```python
from build123d import *

# Parameters (mm, degrees)
F2_SIZE = 2
F3_R    = 5


with BuildPart() as f1:
    # F0 (on Front) → F1 (revolve)
    with BuildSketch(Plane.XZ):
        Polygon((8, 145), (0, 145), (0, 0), (45, 0), (45, 12), (8, 19.864593), align=None)
    revolve(axis=Axis((0, 0, 72.5), (0, 0, 1)))

    # F2
    f2_edges = [f1.edges().sort_by_distance(p)[0] for p in [
        (-8, 0, 145),
    ]]
    chamfer(f2_edges, length=F2_SIZE)

    # F3
    f3_edges = [f1.edges().sort_by_distance(p)[0] for p in [
        (-8, 0, 19.864593),
    ]]
    fillet(f3_edges, radius=F3_R)


solid = f1.part
```
Check sheet for the modelled part. Datum: model origin and axes. Units: mm. A direction names the side the tool comes from. Round coordinates to 2 decimals unless told otherwise and drop trailing zeros. Loops run counter-clockwise (first coordinate to the right, second up) from the corner with the lowest first, then second, coordinate; pieces in that order, holes last. Notation, with made-up numbers: M -2,48.25 L 4,48.25 A16 ccw 4,60.25 Z; hole C 34,13 d3. An arc over 180 degrees is marked long. Answer as a JSON object with one key per item and string values.
1. Access from +Z, -Z, +X, -X, +Y, -Y to the whole of each face (thin tool, end or side, straight path). Record for faces 1 (the cylindrical face through (20.765, -39.923, 6.084)), 2 (the cylindrical face through (-1.73, -7.81, 84.29)).
Reply:
{"face 1": "+Z, -Z", "face 2": "+Z"}
2. Gauge pin test, flat ends, axial feed: P1, Ø1, axis at x = 6.5, y = 9.5, coming from the +Z side; P2, Ø10, axis at x = -2, z = 113, coming from the -Y side; P3, Ø10, axis at x = 10, z = 97, coming from the -Y side (3 decimals). Record the tip position at first contact, or that the pin passes through.
Reply:
{"P1": "stops at z = 19.33", "P2": "stops at y = -8", "P3": "stops at y = -6.245"}
3. Scan lines: line 1 (Z direction, x = -4.5, y = 29); line 2 (Y direction, x = -30, z = 10); line 3 (Y direction, x = 3, z = 31). Record each from-to range of solid material in increasing order.
Reply:
{"line 1": "z = 0 to 15.33", "line 2": "y = -33.54 to 33.54", "line 3": "y = -7.42 to 7.42"}
4. Section check A-A (z = 100.5). Record the boundary of the cut face in (x, y), plus the area to 3 significant figures.
Reply:
{"outline": "C 0,0 d16", "area": "201 mm²"}
